```python
from build123d import *

# Parameters (mm, degrees)
F0_W      = 1.5
F0_H      = 2.5
F1_DEPTH  = 12
F2_R      = 3.5
F3_DEPTH  = 22.5
F4_R      = 10
F5_R      = 2.49999
F6_R      = 1.24999
F7_W      = 12.5
F7_H      = 3.75
F8_DEPTH  = 12
F10_DEPTH = 2.5


# Not quite as in the source:
# - a fillet or chamfer is up to 0.001 mm smaller than in the source, because OpenCascade refuses the exact size


with BuildPart() as f1:
    # F0 (on Top) → F1 (new body)
    with BuildSketch(Plane.XY):
        with BuildLine():
            ThreePointArc((11.25, 0), (10.6066017178, -3.75), (8.75, -7.0710678119))
            Line((8.75, -7.0710678119), (8.75, -10.6066017178))
            ThreePointArc((8.75, -10.6066017178), (10.0907742727, -9.3401699437), (11.25, -7.9056941504))
            Line((11.25, -7.9056941504), (11.25, 0))
        make_face()
        with BuildLine():
            ThreePointArc((-11.25, 0), (0, 11.25), (11.25, 0))
            Line((11.25, 0), (11.25, -7.9056941504))
            ThreePointArc((11.25, -7.9056941504), (13.748354024, 0.2127478073), (11, 8.25))
            ThreePointArc((11, 8.25), (0, 13.75), (-11, 8.25))
            ThreePointArc((-11, 8.25), (-13.748354024, 0.2127478073), (-11.25, -7.9056941504))
            Line((-11.25, -7.9056941504), (-11.25, 0))
        make_face()
        with BuildLine():
            ThreePointArc((11.25, -7.9056941504), (10.0907742727, -9.3401699437), (8.75, -10.6066017178))
            Line((8.75, -10.6066017178), (8.75, -21.9056941504))
            Line((8.75, -21.9056941504), (11.25, -21.9056941504))
            Line((11.25, -21.9056941504), (11.25, -7.9056941504))
        make_face()
        with BuildLine():
            ThreePointArc((-8.75, -7.0710678119), (-10.6066017178, -3.75), (-11.25, 0))
            Line((-11.25, 0), (-11.25, -7.9056941504))
            ThreePointArc((-11.25, -7.9056941504), (-10.0907742727, -9.3401699437), (-8.75, -10.6066017178))
            Line((-8.75, -10.6066017178), (-8.75, -7.0710678119))
        make_face()
        with BuildLine():
            ThreePointArc((-8.75, -10.6066017178), (-10.0907742727, -9.3401699437), (-11.25, -7.9056941504))
            Line((-11.25, -7.9056941504), (-11.25, -21.9056941504))
            Line((-11.25, -21.9056941504), (-8.75, -21.9056941504))
            Line((-8.75, -21.9056941504), (-8.75, -10.6066017178))
        make_face()
        with BuildLine():
            ThreePointArc((-11, 8.25), (0, 13.75), (11, 8.25))
            ThreePointArc((11, 8.25), (10.527864045, 13.4860679775), (15, 16.25))
            Line((15, 16.25), (-15, 16.25))
            ThreePointArc((-15, 16.25), (-10.527864045, 13.4860679775), (-11, 8.25))
        make_face()
        Polygon((-15, 16.25), (15, 16.25), (64.5, 16.25), (64.5, 18.75), (0, 18.75), (-64.5, 18.75), (-64.5, 23.15), (-64.5, 25.65), (-64.5, 30.05), (-67, 30.05), (-67, 16.25), (-64.5, 16.25), align=None)
        Polygon((64.5, 18.75), (64.5, 16.25), (67, 16.25), (67, 30.05), (64.5, 30.05), align=None)
        Polygon((62, 30.05), (64.5, 30.05), (67, 30.05), (67, 32.55), (62, 32.55), align=None)
        Polygon((-67, 32.55), (-67, 30.05), (-64.5, 30.05), (-57.5, 30.05), (-57.5, 32.55), align=None)
        with Locations((-63.75, 24.4)):
            Rectangle(F0_W, F0_H)
    extrude(amount=F1_DEPTH)

    # F2 (on face) → F3 (cut, through all)
    with BuildSketch(Plane(origin=(-11.25, 0, 0), x_dir=(0, -1, 0), z_dir=(-1, 0, 0))):
        with Locations((14.9056941504, 6)):
            Circle(F2_R)
    extrude(amount=-F3_DEPTH, mode=Mode.SUBTRACT)

    # F4
    f4_edges = [f1.edges().sort_by_distance(p)[0] for p in [
        (-8.75, -7.071068, 6),
        (8.75, -7.071068, 6),
        (-11.25, -7.905694, 6),
        (11.25, -7.905694, 6),
    ]]
    fillet(f4_edges, radius=F4_R)

    # F5 (radius 2.5 in the source; OpenCascade refuses exactly that, so slightly less here)
    f5_edges = [f1.edges().sort_by_distance(p)[0] for p in [
        (-57.5, 30.05, 6),
        (-8.75, -21.905694, 6),
        (8.75, -21.905694, 6),
    ]]
    fillet(f5_edges, radius=F5_R)

    # F6 (radius 1.25 in the source; OpenCascade refuses exactly that, so slightly less here)
    f6_edges = [f1.edges().sort_by_distance(p)[0] for p in [
        (-67, 32.55, 6),
        (-67, 16.25, 6),
        (67, 16.25, 6),
        (-63, 23.15, 6),
        (-63, 25.65, 6),
        (62, 32.55, 6),
        (62, 30.05, 6),
        (67, 32.55, 6),
    ]]
    fillet(f6_edges, radius=F6_R)

    # F7 (on face) → F8 (cut, through all)
    with BuildSketch(Plane.XY.offset(12)):
        with Locations((0, 16.875)):
            Rectangle(F7_W, F7_H)
    extrude(amount=-F8_DEPTH, mode=Mode.SUBTRACT)

    # F9 (on face) → F10 (cut, through all)
    with BuildSketch(Plane(origin=(0, 32.55, 0), x_dir=(-1, 0, 0), z_dir=(0, 1, 0))):
        with BuildLine():
            Line((57.5, 12), (57.5, 0))
            ThreePointArc((57.5, 0), (59.1076951546, 6), (57.5, 12))
        make_face()
    extrude(amount=-F10_DEPTH, mode=Mode.SUBTRACT)


solid = f1.part
```
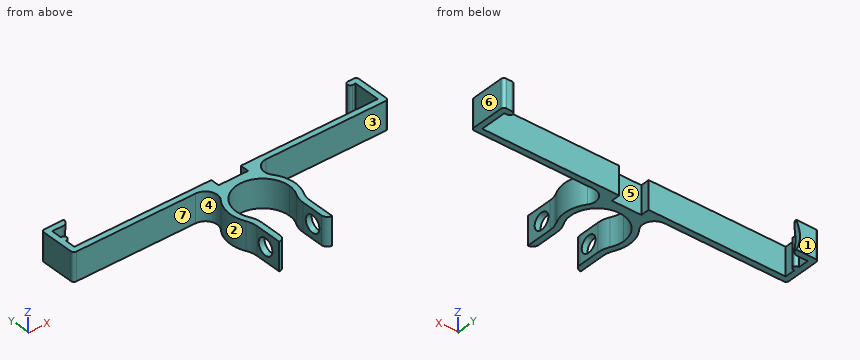
Work out the finished part from the listing and answer in its coordinate system (mm). Face numbers are marked on the shaded views. A direction names the side the tool comes from. Give positions to 0.01 mm unless a question says otherwise; leave off trailing zeros. Write each loop counter-clockwise with the first axis right and the second up, starting at its lowest first coordinate (ties: lowest second). Pieces come first, ordered by that corner, then holes. Notation, with made-up numbers: (83.25, 59.5) - (137.25, 59.5) arc R13 cw to (137.25, 77.5) - close; hole circle Ø1 at (-22.75, 39.5). An arc over 180 degrees is marked (long way). Use one line per item in the form item = value.
1. A cutting plane is placed at D-D (x = -21.5). Write down the section's boundary in (y, z).
Filled in:
outline = (16.25, 0) - (18.75, 0) - (18.75, 12) - (16.25, 12) - close
2. Consider L1, parallel to X at y = 27, z = 7.5; L2, parallel to X at y = 18.5, z = 6; L3, parallel to Y at x = 33.5, z = 3.25. Determine where each line is inside the solid, lowest interval first.
Filled in:
L1 = -67 to -64.5, 64.5 to 67
L2 = -67 to -6.25, 6.25 to 67
L3 = 16.25 to 18.75
3. A cutting plane is placed at A-A (y = 21). Write down the section's boundary in (x, z), and give its area (3 significant figures).
Filled in:
outline = (-67, 0) - (-64.5, 0) - (-64.5, 12) - (-67, 12) - close; (64.5, 0) - (67, 0) - (67, 12) - (64.5, 12) - close
area = 60.0 mm^2
4. For the marked faces 5, 6 and 7, determine the directions among +Z, -Z, +X, -X, +Y, -Y from which every point of the face is accessible in a straight line to the end or side of a thin tool.
Filled in:
face_5 = +Z, -Z, +Y
face_6 = +Z, -Z, +X, +Y, -Y
face_7 = +Z, -Z, -X, -Y
5. A cutting plane is placed at B-B (z = 6). State how many separate pieces and enclosed holes the cut face has, and give its area (3 significant figures).
Filled in:
separate_pieces = 3
enclosed_holes = 0
area = 638 mm^2
6. A cutting plane is placed at C-C (x = 0). Write down the section's boundary in (y, z).
Filled in:
outline = (11.25, 0) - (15, 0) - (15, 12) - (11.25, 12) - close
7. Determine the mould class of the marked faces 1, 2, 3 and 4 for opening direction Y: released by +Y, released by -Y, zero draft, split by the parting line, or undercut.
Filled in:
face_1 = released by +Y
face_2 = undercut
face_3 = released by -Y
face_4 = undercut
8. Each of these flat-tipped pins is pushed along its axis until it touches: pin 1 Ø1.5 at (x, z) = (-6.5, 9.5) entering from +Y; pin 2 Ø3.5 at (x, z) = (-52.5, 8) entering from -Y; pin 3 Ø1 at (y, z) = (-7.5, 9.5) entering from +X. Where does it stop, or does it pass through?
Filled in:
pin_1 = 18.75
pin_2 = 16.25
pin_3 = 11.92
